Work out the finished part from the listing and answer in its coordinate system (mm). A direction names the side the tool comes from. Round coordinates to 2 decimals unless told otherwise and drop trailing zeros. Order: outer loops, then holes, each group sorted by start corner. A loop starts at its lowest first (then second) coordinate and runs counter-clockwise, first axis right, second up. Notation, with made-up numbers: (65.25, 21.25) -> (123.25, 21.25) arc R21 cw to (123.25, 44.25) -> close; hole circle Ø6 at (61, 59). An arc over 180 degrees is marked (long way). Use one line per item in the form item = value.
```python
from build123d import *

# Parameters (mm, degrees)
BOSS_EXTRUDE2_DEPTH       = 72.39
BOSS_EXTRUDE3_DEPTH       = 51.39
F_3_0MM_DOWEL_HOLE1_D     = 3
F_3_0MM_DOWEL_HOLE1_DEPTH = 10
F_3_0MM_DOWEL_HOLE1_TIP   = 0.901290929
F_3_0MM_DOWEL_HOLE2_D     = 3
F_3_0MM_DOWEL_HOLE2_DEPTH = 20
F_3_0MM_DOWEL_HOLE2_TIP   = 0.901290929


with BuildPart() as part:
    # Sketch1 → Boss-Extrude2 (new body)
    with BuildSketch(Plane(origin=(0, 0, 0), x_dir=(1, 0, 0), z_dir=(0, 1, 0))):
        with BuildLine():
            Line((-11.1466884, 31.204775661), (-11.1466884, 17.698170271))
            Line((-11.1466884, 17.698170271), (6.528311604, 17.698170271))
            Line((6.528311604, 17.698170271), (6.528311604, 18.704783117))
            ThreePointArc((6.528311604, 18.704783117), (-2.30169594, 22.370769261), (-5.958035446, 31.204775661))
            Line((-5.958035446, 31.204775661), (-11.1466884, 31.204775661))
        make_face()
        Polygon((-11.1466884, 17.698170271), (-23.8485284, 17.698170271), (-23.8485284, 14.523170271), (6.528311604, 14.523170271), (6.528311604, 17.698170271), align=None)
        with BuildLine():
            Line((6.528311604, 18.704783117), (6.528311604, 17.698170271))
            Line((6.528311604, 17.698170271), (24.2033116, 17.698170271))
            Line((24.2033116, 17.698170271), (24.2033116, 31.204775661))
            Line((24.2033116, 31.204775661), (19.041964554, 31.204775661))
            ThreePointArc((19.041964554, 31.204775661), (15.375970954, 22.361115166), (6.528311604, 18.704783117))
        make_face()
        Polygon((24.2033116, 17.698170271), (6.528311604, 17.698170271), (6.528311604, 14.523170271), (36.9033116, 14.523170271), (36.9033116, 17.698170271), align=None)
    extrude(amount=BOSS_EXTRUDE2_DEPTH)

    # Sketch1_16 → Boss-Extrude3 (add)
    with BuildSketch(Plane(origin=(0, 0, 0), x_dir=(1, 0, 0), z_dir=(0, 1, 0))):
        with BuildLine():
            Line((-5.958035446, 31.204775661), (-5.658035446, 31.204775661))
            ThreePointArc((-5.658035446, 31.204775661), (6.541964554, 19.004775661), (18.741964554, 31.204775661))
            Line((18.741964554, 31.204775661), (19.041964554, 31.204775661))
            ThreePointArc((19.041964554, 31.204775661), (6.541964554, 18.704775661), (-5.958035446, 31.204775661))
        make_face()
    extrude(amount=BOSS_EXTRUDE3_DEPTH)

    # 3.0mm Dowel Hole1
    with Locations(Plane(origin=(0, 0, -17.698170271), x_dir=(-1, 0, 0), z_dir=(0, 0, -1))):
        with Locations((-30.5533116, 66.04), (-30.5533116, 6.35), (17.4985284, 6.35), (17.4985284, 66.04)):
            Hole(F_3_0MM_DOWEL_HOLE1_D / 2, depth=F_3_0MM_DOWEL_HOLE1_DEPTH)
            with Locations((0, 0, -(F_3_0MM_DOWEL_HOLE1_DEPTH + F_3_0MM_DOWEL_HOLE1_TIP / 2))):  # 118° drill point
                Cone(0, F_3_0MM_DOWEL_HOLE1_D / 2, F_3_0MM_DOWEL_HOLE1_TIP, mode=Mode.SUBTRACT)

    # 3.0mm Dowel Hole2
    with Locations(Plane(origin=(0, 0, -31.204775661), x_dir=(-1, 0, 0), z_dir=(0, 0, -1))):
        with Locations((-21.6233116, 66.04), (-21.6233116, 6.35), (8.5666884, 6.35), (8.5666884, 66.04)):
            Hole(F_3_0MM_DOWEL_HOLE2_D / 2, depth=F_3_0MM_DOWEL_HOLE2_DEPTH)
            with Locations((0, 0, -(F_3_0MM_DOWEL_HOLE2_DEPTH + F_3_0MM_DOWEL_HOLE2_TIP / 2))):  # 118° drill point
                Cone(0, F_3_0MM_DOWEL_HOLE2_D / 2, F_3_0MM_DOWEL_HOLE2_TIP, mode=Mode.SUBTRACT)


solid = part.part
```
Item 1: The part is cut by section B-B, the plane z = -26.5. Give the vertices of the cut face in (x, y), and give its area (3 significant figures).
Findings:
outline = (-11.15, 0) -> (-4.71, 0) -> (-4.71, 51.39) -> (-5.04, 51.39) -> (-5.04, 72.39) -> (-11.15, 72.39) -> close; (17.8, 0) -> (24.2, 0) -> (24.2, 72.39) -> (18.12, 72.39) -> (18.12, 51.39) -> (17.8, 51.39) -> close; hole circle Ø3 at (-8.57, 6.35); hole circle Ø3 at (-8.57, 66.04); hole circle Ø3 at (21.62, 6.35); hole circle Ø3 at (21.62, 66.04)
area = 887 mm^2
Item 2: The part is cut by section C-C, the plane y = 45. Give the vertices of the cut face in (x, z).
Findings:
outline = (-23.85, -17.7) -> (-11.15, -17.7) -> (-11.15, -31.2) -> (-5.66, -31.2) arc R12.2 cw to (18.74, -31.2) -> (24.2, -31.2) -> (24.2, -17.7) -> (36.9, -17.7) -> (36.9, -14.52) -> (-23.85, -14.52) -> close
Item 3: The part is cut by section D-D, the plane y = 6.35. Give the vertices of the cut face in (x, z).
Findings:
outline = (-23.85, -17.7) -> (-19, -17.7) -> (-19, -14.52) -> (-23.85, -14.52) -> close; (-16, -17.7) -> (-11.15, -17.7) -> (-11.15, -31.2) -> (-10.07, -31.2) -> (-10.07, -14.52) -> (-16, -14.52) -> close; (-7.07, -31.2) -> (-5.66, -31.2) arc R12.2 cw to (18.74, -31.2) -> (20.12, -31.2) -> (20.12, -14.52) -> (-7.07, -14.52) -> close; (23.12, -31.2) -> (24.2, -31.2) -> (24.2, -17.7) -> (29.05, -17.7) -> (29.05, -14.52) -> (23.12, -14.52) -> close; (32.05, -17.7) -> (36.9, -17.7) -> (36.9, -14.52) -> (32.05, -14.52) -> close
Item 4: Determine the mould class of faces 4 (the cylindrical face through (6.274, 25.335, -19.008)), 5 (the cylindrical face through (-7.76, 67.305, -22.747)), 6 (the cylindrical face through (31.36, 67.305, -16.088)), 7 (the flat face through (7, 0, -17)) for opening direction Y: released by +Y, released by -Y, zero draft, split by the parting line, or undercut.
Findings:
face_4 = zero draft
face_5 = undercut
face_6 = undercut
face_7 = released by -Y
Item 5: The part is cut by section A-A, the plane y = 66.04. Give the vertices of the cut face in (x, z), and give its area (3 significant figures).
Findings:
outline = (-23.85, -17.7) -> (-19, -17.7) -> (-19, -14.52) -> (-23.85, -14.52) -> close; (-16, -17.7) -> (-11.15, -17.7) -> (-11.15, -31.2) -> (-10.07, -31.2) -> (-10.07, -14.52) -> (-16, -14.52) -> close; (-7.07, -31.2) -> (-5.96, -31.2) arc R12.5 cw to (19.04, -31.2) -> (20.12, -31.2) -> (20.12, -14.52) -> (-7.07, -14.52) -> close; (23.12, -31.2) -> (24.2, -31.2) -> (24.2, -17.7) -> (29.05, -17.7) -> (29.05, -14.52) -> (23.12, -14.52) -> close; (32.05, -17.7) -> (36.9, -17.7) -> (36.9, -14.52) -> (32.05, -14.52) -> close
area = 306 mm^2
Item 6: Flat-ended cylindrical pins translate along their axes: P1, Ø1.5, axis at y = 30, z = -28, coming from the -X side; P2, Ø3.5, axis at x = 30.55, y = 66.04, coming from the -Z side; P3, Ø7, axis at y = 49.5, z = -23.5, coming from the +X side. Find the tip coordinate at first contact, or state that the pin passes through.
Findings:
P1 = -11.15
P2 = -17.7
P3 = 24.2
Item 7: Consider line 1 along X through (y, z) = (66.04, -16.9); line 2 along Y through (x, z) = (22, -16.5); line 3 along Z through (x, y) = (24.5, 47.5). Determine where each line is inside the solid, lowest interval first.
Findings:
line_1 = -23.85 to -19, -16 to -10.07, -7.07 to 20.12, 23.12 to 29.05, 32.05 to 36.9
line_2 = 0 to 4.9, 7.8 to 64.59, 67.49 to 72.39
line_3 = -17.7 to -14.52
Item 8: For faces 1 (the flat face through (31, 36, -17.698)), 2 (the flat face through (-17, 36, -17.698)), 3 (the cylindrical face through (22.43, 67.305, -22.747)), determine the directions among +Z, -Z, +X, -X, +Y, -Y from which every point of the face is accessible in a straight line to the end or side of a thin tool.
Findings:
face_1 = -Z, +X, +Y, -Y
face_2 = -Z, -X, +Y, -Y
face_3 = +Z, -Z
